For this review, take the finished solid that the model builds, in its own axes (mm). Coordinates: 2 decimals unless noted, no trailing zeros. Write each loop counter-clockwise with the first axis right and the second up, starting at its lowest first coordinate (ties: lowest second). Pieces come first, ordered by that corner, then holes.
1) To check wall thickness, follow line 1 along Y through (x, z) = (-9.2, -36.75); line 2 along Z through (x, y) = (-8.9, 43); line 3 along Z through (x, y) = (-9.25, 20). State the ranges of each line that lie inside material, in increasing order.
2) Mouldability with a two-part tool opening along Y and no side actions: class faces 1 (the face through (-9.24, 44.33, -68.19)), 2 (the face through (-8.32, -72.71, -36.9)), 3 (the face through (-8, 22, 0)), 4 (the face through (-8.28, 46.1, -72.64)) as pulls with the +Y half, pulls with the -Y half, needs draft (parallel to the pull), parting line crosses it, or undercut.
3) We need section A-A on z = -36.75. Write out the cut boundary in (x, y).
4) We need section B-B on x = -9.3. Give the number of separate pieces and of enclosed holes in the cut face, then the cut area to 3 significant figures.
Autodesk Inventor part; units mm, degrees
ref_plane "Work Plane1" through (-9.8, 47, 0) normal (0.7071, 0.7071, 0) x (0, 0, -1)
ref_plane "CentrePlane" through (8, 0, 0) normal (1, 0, 0) x (0, 0, -1)
ref_plane "YZ Plane" through (0, 0, 0) normal (1, 0, 0) x (0, 1, 0)
sketch "Sketch1" plane through (0, 0, 0) normal (0, 0, 1) x (1, 0, 0)
  line L0 (0, 0) -> (16, 0) construction
  line L1 (16, 0) -> (16, 8) construction
  line L2 (0, 8) -> (0, 0) construction
  line L3 (5.5, 10.5) -> (0, 10.5) construction
  line L4 (0, 10.5) -> (0, 8) construction
  line L5 (13.5, 10.5) -> (16, 10.5) construction
  line L6 (16, 10.5) -> (16, 8) construction
  line L7 (6.5, 37) -> (12.5, 37) construction
  line L8 (12.5, 37) -> (12.5, 8) construction
  line L9 (12.5, 8) -> (6.5, 8) construction
  line L10 (6.5, 8) -> (6.5, 37) construction
  line L11 (0.5, 34.5) -> (15.5, 34.5) construction
  line L12 (15.5, 34.5) -> (15.5, 10.5) construction
  line L13 (15.5, 10.5) -> (0.5, 10.5) construction
  line L14 (0.5, 10.5) -> (0.5, 34.5) construction
  line L15 (-6.8, 0) -> (-6.8, 39)
  line L16 (-6.8, 39) -> (22.8, 39)
  line L17 (8, -29.8106) -> (8, -55.1885) construction
  line L18 (-9.8, 47) -> (-9.8, 0)
  line L19 (-6.8, 0) -> (-9.8, 0)
  line L20 (-9.8, 47) -> (10, 47)
  line L21 (25.8, 47) -> (25.8, 0)
  line L22 (22.8, 0) -> (25.8, 0)
  line L23 (25.8, 47) -> (10, 47)
  line L24 (22.8, 0) -> (22.8, 39)
  line L25 (16.05, 25.6) -> (16.05, 19.4) construction
  line L26 (-0.05, 19.4) -> (-0.05, 25.6) construction
  line L27 (-0.05, 25.6) -> (0.5, 25.6) construction
  line L28 (16.05, 25.6) -> (15.5, 25.6) construction
  line L29 (16.05, 19.4) -> (15.5, 19.4) construction
  line L30 (-0.05, 19.4) -> (0.5, 19.4) construction
  line L31 (16.05, 22.5) -> (-0.05, 22.5) construction
  line L32 (0, 8) -> (16, 8) construction
  line L33 (5.5, 10.5) -> (5.5, 8) construction
  line L34 (13.5, 10.5) -> (13.5, 8) construction
  line L35 (5.5, 8) -> (13.5, 8) construction
  point P0 (6.5, 22.5)
  point P1 (0.5, 22.5)
  point P2 (9.5, 8)
  point P3 (8, 0)
  point P4 (8, 39)
  point P5 (8, -42.4996)
  point P6 (9.5, 8)
  point P7 (8, 22.5)
  dimension "d1" = 16
  dimension "d7" = 6
  dimension "d9" = 6
  dimension "d10" = 3
  dimension "d11" = 29
  dimension "d12" = 24
  dimension "d19" = 29.6
  dimension "d20" = 2
  dimension "thickness" = 3
  dimension "d23" = 8
  dimension "d31" = 22.5
  dimension "d40" = 24.5
  dimension "d41" = 39
  dimension "d60" = 6.2
  dimension "d62" = 16.1
  dimension "d63" = 8
  dimension "d64" = 8
  dimension "d65" = 1
  dimension "d66" = 2.5
extrude "LENGTH" add sketch "Sketch1" against normal blind 73.5
sketch "Sketch2" plane through (-9.8, 0, 0) normal (-1, 0, 0) x (0, 0, 1)
  circle A0 centre (-12, 22.5) radius 3
  circle A1 centre (-61.5, 22.5) radius 3
  line L0 (-73.5, 0) -> (-73.5, 47) construction
  line L1 (0, 47) -> (0, 0) construction
  dimension "d26" = 6
  dimension "d28" = 6
  dimension "d29" = 12
  dimension "d30" = 12
  dimension "d32" = 22.5
extrude "Extrusion2" cut sketch "Sketch2" against normal through all
ref_plane "Work Plane1" through (-9.8, 47, 0) normal (0.7071, 0.7071, 0) x (0, 0, -1)
ref_plane "CentrePlane" through (8, 0, 0) normal (1, 0, 0) x (0, 0, -1)
sketch "Measurements" plane through (-9.8, 0, 0) normal (-1, 0, 0) x (0, 0, 1)
  line L0 (-18.9044, 8) -> (-18.9044, 0) construction
  line L1 (0, 0) -> (0, 8) construction
  spline S0 degree 3 poles (-18.9044, 0) (-18.8729, 0.004) (-18.7747, 0.0145) (-18.6089, 0.0198) (-18.4076, 0.0173) (-18.2077, -0.0064) (-18.0095, -0.0413) (-17.7511, -0.1137) (-17.4304, -0.2111) (-17.1073, -0.2999) (-16.8501, -0.3765) (-16.6638, -0.4528) (-16.4821, -0.5394) (-16.3106, -0.6447) (-16.1439, -0.7575) (-15.9893, -0.8866) (-15.8435, -1.0251) (-15.7068, -1.1728) (-15.5834, -1.3319) (-15.4695, -1.4977) (-15.3662, -1.6705) (-15.2464, -1.9105) (-15.1208, -2.2219) (-15.0142, -2.6104) (-14.9462, -3.0072) (-14.9104, -3.408) (-14.9034, -3.8104) (-14.9258, -4.2123) (-14.9692, -4.6123) (-15.0344, -5.0094) (-15.0913, -5.2714) (-15.1198, -5.4024) knots -0.847201 -0.847201 -0.847201 -0.847201 -0.83705 -0.815587 -0.794126 -0.772659 -0.751201 -0.729734 -0.686802 -0.64387 -0.622403 -0.600945 -0.579478 -0.558017 -0.536554 -0.515088 -0.49363 -0.472163 -0.450698 -0.429238 -0.407769 -0.386302 -0.343394 -0.300476 -0.257562 -0.214646 -0.17172 -0.12879 -0.085861 -0.04293 0 0 0 0 construction
  spline S1 degree 3 poles (-4.5152, -5.4024) (-4.5336, -5.2605) (-4.5704, -4.9766) (-4.6037, -4.5484) (-4.6135, -4.119) (-4.6009, -3.6896) (-4.557, -3.2623) (-4.4825, -2.8392) (-4.3742, -2.4233) (-4.2256, -2.0199) (-4.0637, -1.7) (-3.9145, -1.4557) (-3.7891, -1.2813) (-3.6528, -1.1153) (-3.5072, -0.9573) (-3.3484, -0.8126) (-3.1807, -0.6785) (-3.0046, -0.5552) (-2.8172, -0.4504) (-2.6251, -0.3539) (-2.424, -0.2783) (-2.219, -0.214) (-1.9385, -0.1559) (-1.5868, -0.0908) (-1.2369, -0.0163) (-0.9555, 0.0373) (-0.7415, 0.0564) (-0.5268, 0.0635) (-0.3125, 0.0479) (-0.1366, 0.0272) (-0.0331, 0.0071) (0, 0) knots -1.373604 -1.373604 -1.373604 -1.373604 -1.330674 -1.287743 -1.244814 -1.201884 -1.158958 -1.116042 -1.073128 -1.03021 -0.987302 -0.965835 -0.944366 -0.922906 -0.901441 -0.879974 -0.858516 -0.83705 -0.815587 -0.794126 -0.772659 -0.751201 -0.729734 -0.686802 -0.64387 -0.622403 -0.600945 -0.579478 -0.558017 -0.536554 -0.526403 -0.526403 -0.526403 -0.526403 construction
  spline S2 degree 3 poles (-7.7374, -14.9236) (-7.6284, -14.7418) (-7.4104, -14.3783) (-7.0987, -13.824) (-6.7983, -13.2636) (-6.5111, -12.6963) (-6.2373, -12.1224) (-5.9778, -11.5419) (-5.7335, -10.9548) (-5.5053, -10.3613) (-5.2945, -9.7613) (-5.1024, -9.1551) (-4.9307, -8.5428) (-4.7815, -7.9246) (-4.6579, -7.3008) (-4.5633, -6.6718) (-4.516, -6.1439) (-4.4999, -5.72) (-4.5101, -5.5083) (-4.5152, -5.4024) knots -1.017256 -1.017256 -1.017256 -1.017256 -0.953675 -0.890094 -0.826513 -0.762932 -0.699351 -0.63577 -0.572189 -0.508609 -0.445029 -0.381449 -0.31787 -0.254291 -0.190714 -0.127139 -0.063568 -0.03178 0 0 0 0 construction
  arc A0 (-11.8976, -14.9236) -> (-7.7374, -14.9236) centre (-9.8175, 41.288) ccw construction
  spline S3 degree 3 poles (-15.1198, -5.4024) (-15.1249, -5.5083) (-15.1352, -5.72) (-15.119, -6.1439) (-15.0717, -6.6718) (-14.9771, -7.3008) (-14.8535, -7.9246) (-14.7043, -8.5428) (-14.5326, -9.1551) (-14.3405, -9.7613) (-14.1297, -10.3613) (-13.9015, -10.9548) (-13.6572, -11.5419) (-13.3977, -12.1224) (-13.1239, -12.6963) (-12.8366, -13.2636) (-12.5363, -13.824) (-12.2245, -14.3782) (-12.0065, -14.7418) (-11.8976, -14.9236) knots -1.017256 -1.017256 -1.017256 -1.017256 -0.985476 -0.953687 -0.890117 -0.826542 -0.762964 -0.699386 -0.635807 -0.572227 -0.508647 -0.445066 -0.381486 -0.317905 -0.254324 -0.190743 -0.127162 -0.063581 0 0 0 0 construction
  line L2 (-18.9044, 8) -> (0, 8) construction
  line L3 (0, 43) -> (0, 0) construction
  circle A1 centre (-9.8175, -59.712) radius 50 construction
  line L4 (0, 0) -> (-73.5, 0)
  point P0 (-9.8175, -14.962)
  dimension "d42" = 8
  dimension "d43" = 100
  dimension "d44" = 44.75
  dimension "d46" = 9.8175
  dimension "d47" = 14.962
  dimension "d49" = 59.712
sketch "Sketch5" plane through (-9.8, 0, 0) normal (-1, 0, 0) x (0, 0, 1)
  circle A0 centre (-36.75, -59.712) radius 50 construction
  line L0 (0, 0) -> (-73.5, 0)
  circle A1 centre (-36.75, -59.712) radius 5
  arc A2 (-46.4124, -68.4091) -> (-27.0876, -68.4091) centre (-36.75, -59.712) ccw
  line L1 (-36.75, 56.2641) -> (-36.75, 80.2382)
  line L2 (0, 0) -> (-73.5, 0)
  spline S0 degree 4 poles (0, 0) (0, -20.6328) (-6.9347, -45.2291) (-15.8528, -55.9272) (-27.0876, -68.4091) knots 0 0 0 0 0 1 1 1 1 1
  line L3 (0, 0) -> (0, 47)
  spline S1 degree 4 poles (-73.5, 0) (-73.5, -20.6328) (-66.5653, -45.2291) (-57.6472, -55.9272) (-46.4124, -68.4091) knots 0 0 0 0 0 1 1 1 1 1
  line L4 (-73.5, 47) -> (-73.5, 0)
  point P0 (-36.75, 0)
  point P1 (-36.75, 0)
  point P2 (-9.7513, -43.7182)
  point P3 (-63.7487, -43.7182)
  dimension "d50" = 59.712
  dimension "d51" = 100
  dimension "bearingOD" = 10
  dimension "d53" = 8
extrude "Extrusion4" add sketch "Sketch5" against normal up to surface (3 mm away)
mirror "Mirror2" about plane through (8, 0, 0) normal (1, 0, 0) of "Extrusion4"
sketch "Sketch6" plane through (-6.8, 39, 0) normal (1, 0, 0) x (0, 0, -1)
  line L0 (-41.9522, 50.4986) -> (119.8165, 50.4986)
  line L1 (119.8165, 50.4986) -> (119.8165, -146.1585)
  line L2 (119.8165, -146.1585) -> (-41.9522, -146.1585)
  line L3 (-41.9522, -146.1585) -> (-41.9522, 50.4986)
  point P0 (0, -39)
extrude "Extrusion5" cut sketch "Sketch6" along normal through all
sketch "Sketch7" plane through (-6.8, 47, 0) normal (1, 0, 0) x (0, 0, -1)
  circle A0 centre (6, -4) radius 3.485
  circle A1 centre (36.75, -24) radius 3.485
  line L0 (36.75, -50.9937) -> (36.75, -60.2424)
  line L1 (0, 0) -> (73.5, 0)
  circle A2 centre (67.5, -4) radius 3.485
  line L2 (0, -47) -> (0, 0)
  point P0 (36.75, 0)
  dimension "d69" = 6.97
  dimension "d70" = 6
  dimension "d71" = 24
  dimension "d72" = 4
hole "Hole1" at (-6.8, 43, -6) at (-6.8, 23, -36.75) at (-6.8, 43, -67.5) direction (-1, 0, 0) diameter 3 end through all countersink diameter 6.72 countersink angle 90
fillet "Fillet3" radius 3 2 edges at (-8.3, 47, 0) (-8.3, 47, -73.5)
equation "\"d23\" = d0"
equation "\"tol\" = 1"
properties part number "trolley6mm-sides"
Result:
1. line 1: y = -72.71 to -64.71, -54.71 to 21.5, 24.5 to 47
1. line 2: z = -73.5 to -69, -66 to -7.5, -4.5 to 0
1. line 3: z = -73.5 to -63.16, -59.84 to -13.66, -10.34 to 0
2. face 1: undercut
2. face 2: pulls with the -Y half
2. face 3: needs draft
2. face 4: pulls with the +Y half
3. outline: (-9.8, -72.71) - (-6.8, -72.71) - (-6.8, -64.71) - (-9.8, -64.71) - close; (-9.8, -54.71) - (-6.8, -54.71) - (-6.8, 19.64) - (-8.66, 21.5) - (-9.8, 21.5) - close; (-9.8, 24.5) - (-8.66, 24.5) - (-6.8, 26.36) - (-6.8, 47) - (-9.8, 47) - close
4. separate pieces: 1
4. enclosed holes: 6
4. area: 7,230 mm2
